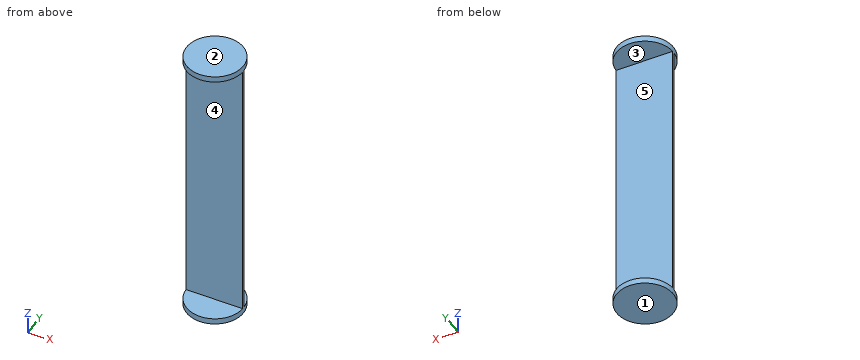
from build123d import *

# Parameters (mm, degrees)
BOSS_EXTRU_2_DEPTH      = 120
BOSS_EXTRU_2_DEPTH_BACK = 120
ESQUISSE1_R             = 24
ESQUISSE2_W             = 230
ESQUISSE2_H             = 23
ENL_V_MAT_EXTRU_1_DEPTH = 125.707658145


with BuildPart() as part:
    # Esquisse1 → Boss.-Extru.2 (new, two sides: drawn at the far end of the back side and taken through both)
    with BuildSketch(Plane.XY.offset(-BOSS_EXTRU_2_DEPTH_BACK)):
        Circle(ESQUISSE1_R)
    extrude(amount=BOSS_EXTRU_2_DEPTH + BOSS_EXTRU_2_DEPTH_BACK)

    # Esquisse2 → Enlèv. mat.-Extru.1 (cut, symmetric)
    with BuildSketch(Plane(origin=(0, 0, 0), x_dir=(0, 0, -1), z_dir=(1, 0, 0))):
        with Locations((0, 12.5)):
            Rectangle(ESQUISSE2_W, ESQUISSE2_H)
    enl_v_mat_extru_1 = extrude(amount=ENL_V_MAT_EXTRU_1_DEPTH, both=True, mode=Mode.SUBTRACT)

    # Symétrie1: Enlèv. mat.-Extru.1 across plane
    add(enl_v_mat_extru_1.mirror(Plane.ZX), mode=Mode.SUBTRACT)


solid = part.part
Geometry check sheet. Reference: the model listing, model coordinates, mm. Face numbers are marked on the shaded views. A direction names the side the tool comes from. Give positions to 0.01 mm unless a question says otherwise; leave off trailing zeros. Order: outer loops, then holes, each group sorted by start corner. A loop starts at its lowest first (then second) coordinate and runs counter-clockwise, first axis right, second up.
1. Sectioned sample at A-A (y = -13). Record the boundary of the cut face in (x, z).
Completed:
outline: (-20.17, -120) - (20.17, -120) - (20.17, -115) - (-20.17, -115) - close; (-20.17, 115) - (20.17, 115) - (20.17, 120) - (-20.17, 120) - close
2. Scan lines: line 1 (Z direction, x = -12, y = -5.5); line 2 (Y direction, x = -11.5, z = 108). Record each from-to range of solid material in increasing order.
Completed:
line 1: z = -120 to -115, 115 to 120
line 2: y = -1 to 1
3. Access from +Z, -Z, +X, -X, +Y, -Y to the whole of each face (thin tool, end or side, straight path). Record for the marked faces 4 and 5.
Completed:
face 4: +X, -X, -Y
face 5: +X, -X, +Y
4. Draft check along Z on the marked faces 1, 2 and 3. Enter one of: pulls with the +Z half, pulls with the -Z half, needs draft (parallel to the pull), parting line crosses it, or undercut.
Completed:
face 1: pulls with the -Z half
face 2: pulls with the +Z half
face 3: undercut
5. Sectioned sample at B-B (x = 0). Record the boundary of the cut face in (y, z).
Completed:
outline: (-24, -120) - (24, -120) - (24, -115) - (1, -115) - (1, 115) - (24, 115) - (24, 120) - (-24, 120) - (-24, 115) - (-1, 115) - (-1, -115) - (-24, -115) - close
6. Sectioned sample at D-D (z = 24.5). Record the boundary of the cut face in (x, y).
Completed:
outline: (-23.98, -1) - (23.98, -1) arc R24 ccw to (23.98, 1) - (-23.98, 1) arc R24 ccw to start
7. Depth check by flat-ended pin: pin 1 (8 mm diameter, centred on x = -13, z = 89, fed in from +Y); pin 2 (10 mm diameter, centred on y = 10.5, z = -81.5, fed in from -X). Enter the tip coordinate at first touch or a pass-through.
Completed:
pin 1: stops at y = 1
pin 2: passes through
8. Sectioned sample at C-C (y = 16). Record the boundary of the cut face in (x, z), then the cut area to 3 significant figures.
Completed:
outline: (-17.89, -120) - (17.89, -120) - (17.89, -115) - (-17.89, -115) - close; (-17.89, 115) - (17.89, 115) - (17.89, 120) - (-17.89, 120) - close
area: 358 mm2
